```python
from build123d import *

# Parameters (mm, degrees)
SKETCH_1_W               = 2800
SKETCH_1_H               = 720
EXTRUDE_1_DEPTH          = 14
SKETCH_5_W               = 980
SKETCH_5_H               = 100
EXTRUDE_2_DEPTH          = 8
SKETCH_9_W               = 980
SKETCH_9_H               = 8
EXTRUDE_3_DEPTH          = 100
MIRROR_4_COPY_1_SKETCH_W = 980
MIRROR_4_COPY_1_SKETCH_H = 100
MIRROR_4_COPY_1_DEPTH    = 8
MIRROR_4_COPY_2_SKETCH_W = 980
MIRROR_4_COPY_2_SKETCH_H = 8
MIRROR_4_COPY_2_DEPTH    = 100
MIRROR_4_COPY_3_SKETCH_W = 980
MIRROR_4_COPY_3_SKETCH_H = 100
MIRROR_4_COPY_3_DEPTH    = 8
SKETCH_11_W              = 240
SKETCH_11_H              = 80
EXTRUDE_4_DEPTH          = 32
SKETCH_12_R              = 13
CUT_EXTRUDE_5_DEPTH      = 1449.999654934
PATTERN_LINEAR_4_COUNT   = 3
PATTERN_LINEAR_4_PITCH   = 80
SKETCH_11_3_W            = 240
SKETCH_11_3_H            = 80
EXTRUDE_6_DEPTH          = 54
MIRROR_8_COPY_1_SKETCH_W = 240
MIRROR_8_COPY_1_SKETCH_H = 80
MIRROR_8_COPY_1_DEPTH    = 54


with BuildPart() as part:
    # Sketch 1 → Extrude 1 (new body)
    with BuildSketch(Plane.XY):
        Rectangle(SKETCH_1_W, SKETCH_1_H)
    extrude(amount=EXTRUDE_1_DEPTH)

    # Sketch 5 → Extrude 2 (add)
    with BuildSketch(Plane.XY.offset(14)):
        with Locations((-490, 310)):
            Rectangle(SKETCH_5_W, SKETCH_5_H)
    extrude_2 = extrude(amount=EXTRUDE_2_DEPTH)

    # Sketch 9 → Extrude 3 (add)
    with BuildSketch(Plane.XY.offset(22)):
        with Locations((-490, 264)):
            Rectangle(SKETCH_9_W, SKETCH_9_H)
    extrude_3 = extrude(amount=EXTRUDE_3_DEPTH)

    # Mirror 3: Extrude 2, Extrude 3 across plane
    add(extrude_2.mirror(Plane.ZX))
    add(extrude_3.mirror(Plane.ZX))

    # Mirror 4: Extrude 3 across plane
    add(extrude_3.mirror(Plane(origin=(0, 0, 0), x_dir=(0, 0, 1), z_dir=(1, 0, 0))))

    # Mirror 4 copy 1 sketch → Mirror 4 copy 1 (add)
    with BuildSketch(Plane(origin=(0, 0, 14), x_dir=(-1, 0, 0), z_dir=(0, 0, 1))):
        with Locations((-490, 310)):
            Rectangle(MIRROR_4_COPY_1_SKETCH_W, MIRROR_4_COPY_1_SKETCH_H)
    extrude(amount=MIRROR_4_COPY_1_DEPTH)

    # Mirror 4 copy 2 sketch → Mirror 4 copy 2 (add)
    with BuildSketch(Plane(origin=(0, 0, 22), x_dir=(-1, 0, 0), z_dir=(0, 0, 1))):
        with Locations((-490, 264)):
            Rectangle(MIRROR_4_COPY_2_SKETCH_W, MIRROR_4_COPY_2_SKETCH_H)
    extrude(amount=MIRROR_4_COPY_2_DEPTH)

    # Mirror 4 copy 3 sketch → Mirror 4 copy 3 (add)
    with BuildSketch(Plane(origin=(0, 0, 14), x_dir=(-1, 0, 0), z_dir=(0, 0, 1))):
        with Locations((-490, -310)):
            Rectangle(MIRROR_4_COPY_3_SKETCH_W, MIRROR_4_COPY_3_SKETCH_H)
    extrude(amount=MIRROR_4_COPY_3_DEPTH)

    # Sketch 11 → Extrude 4 (add)
    with BuildSketch(Plane.XY.offset(22)):
        with Locations((-250, 308)):
            Rectangle(SKETCH_11_W, SKETCH_11_H)
    extrude(amount=-EXTRUDE_4_DEPTH)

    # Sketch 12 → Cut-Extrude 5 (cut, through all)
    with BuildSketch(Plane.XY.offset(22)):
        with Locations((-330, 304)):
            Circle(SKETCH_12_R)
    cut_extrude_5 = extrude(amount=-CUT_EXTRUDE_5_DEPTH, mode=Mode.SUBTRACT)

    # Pattern Linear 4: Cut-Extrude 5 ×3
    with Locations(*[(i * PATTERN_LINEAR_4_PITCH, 0, 0) for i in range(1, PATTERN_LINEAR_4_COUNT)]):
        add(cut_extrude_5, mode=Mode.SUBTRACT)

    # Sketch 11_3 → Extrude 6 (add)
    with BuildSketch(Plane.XY.offset(22)):
        with Locations((-250, 308)):
            Rectangle(SKETCH_11_3_W, SKETCH_11_3_H)
    extrude_6 = extrude(amount=-EXTRUDE_6_DEPTH)

    # Mirror 7: Extrude 6 across plane
    add(extrude_6.mirror(Plane.ZX))

    # Mirror 8: Extrude 6 across plane
    add(extrude_6.mirror(Plane(origin=(0, 0, 0), x_dir=(0, 0, 1), z_dir=(1, 0, 0))))

    # Mirror 8 copy 1 sketch → Mirror 8 copy 1 (add)
    with BuildSketch(Plane(origin=(0, 0, 22), x_dir=(-1, 0, 0), z_dir=(0, 0, 1))):
        with Locations((-250, 308)):
            Rectangle(MIRROR_8_COPY_1_SKETCH_W, MIRROR_8_COPY_1_SKETCH_H)
    extrude(amount=-MIRROR_8_COPY_1_DEPTH)


solid = part.part
```
Input: part model. Units: mm. Frame: model coordinates. A direction names the side the tool comes from. Round coordinates to 2 decimals unless told otherwise and drop trailing zeros. Loops run counter-clockwise (first coordinate to the right, second up) from the corner with the lowest first, then second, coordinate; pieces in that order, holes last.
1) Section query B-B on x = -263. Return the cut outline in (y, z), plus the area to 3 significant figures.
Ans:
outline: (-360, 0) - (-348, 0) - (-348, -32) - (-268, -32) - (-268, 0) - (268, 0) - (268, -32) - (348, -32) - (348, 0) - (360, 0) - (360, 22) - (268, 22) - (268, 122) - (260, 122) - (260, 14) - (-260, 14) - (-260, 122) - (-268, 122) - (-268, 22) - (-360, 22) - close
area: 18,400 mm2
2) Section query A-A on z = 90.5. Return the cut outline in (x, y), plus the area to 3 significant figures.
Ans:
outline: (-980, -268) - (980, -268) - (980, -260) - (-980, -260) - close; (-980, 260) - (980, 260) - (980, 268) - (-980, 268) - close
area: 31,400 mm2
3) Section query C-C on y = 85. Return the cut outline in (x, z).
Ans:
outline: (-1400, 0) - (1400, 0) - (1400, 14) - (-1400, 14) - close
4) Material intervals for line 1 (Y direction, x = 726.5, z = 74); line 2 (Y direction, x = 297, z = -18); line 3 (Z direction, x = 1072.5, y = -176), sorted ascending.
Ans:
line 1: y = -268 to -260, 260 to 268
line 2: y = -348 to -268, 268 to 348
line 3: z = 0 to 14
5) Pin query (flat end, axial travel): pin 1 (16 mm diameter, centred on x = 230.5, z = -17.5, fed in from +Y); pin 2 (9.5 mm diameter, centred on y = -307.5, z = -21, fed in from -X); pin 3 (1 mm diameter, centred on x = 816, y = -19, fed in from -Z). Return the tip coordinate at first contact, or that it passes through.
Ans:
pin 1: stops at y = 348
pin 2: stops at x = -370
pin 3: stops at z = 0
6) Set-up query: faces 1 (the flat face through (980, -265, 44)), 2 (the flat face through (-980, 265, 44)), 3 (the flat face through (14, -260, 67)). Return all of +Z, -Z, +X, -X, +Y, -Y with unobstructed straight access to the full face (end or side cutting, diameter ignored); none if empty.
Ans:
face 1: +Z, +X, +Y, -Y
face 2: +Z, -X, +Y, -Y
face 3: +Z, +X, -X
7) Pull-direction query (Y, two-part tool) for faces 4 (the flat face through (14, -315, 22)), 5 (the flat face through (14, 268, 71)), 6 (the flat face through (-20, 5, 0)); classes: released by +Y, released by -Y, zero draft, split by the parting line, or undercut.
Ans:
face 4: zero draft
face 5: released by +Y
face 6: undercut
8) Section query D-D on x = -606. Return the cut outline in (y, z).
Ans:
outline: (-360, 0) - (360, 0) - (360, 22) - (268, 22) - (268, 122) - (260, 122) - (260, 14) - (-260, 14) - (-260, 122) - (-268, 122) - (-268, 22) - (-360, 22) - close
